from build123d import *

# Parameters (mm, degrees)
F0_W     = 98.428418
F0_H     = 58.695849
F1_DEPTH = 38.1
F2_W     = 23.026837
F2_H     = 29.122172
F3_DEPTH = 37.592
F4_W     = 26.407606
F4_H     = 29.122172
F5_DEPTH = 37.338
F6_W     = 98.428428
F6_H     = 23.929847
F7_DEPTH = 119.888


with BuildPart() as f1:
    # F0 (on Front) → F1 (new body)
    with BuildSketch(Plane.XZ):
        with Locations((-0.45151, 0.225753)):
            Rectangle(F0_W, F0_H)
    extrude(amount=F1_DEPTH)

    # F2 (on face) → F3 (join)
    with BuildSketch(Plane.XZ.offset(38.1)):
        with Locations((-38.1523, -14.561086)):
            Rectangle(F2_W, F2_H)
    extrude(amount=F3_DEPTH)

    # F4 (on face) → F5 (join)
    with BuildSketch(Plane.XZ.offset(38.1)):
        with Locations((35.558896, -14.561086)):
            Rectangle(F4_W, F4_H)
    extrude(amount=F5_DEPTH)

    # F6 (on Front) → F7 (join)
    with BuildSketch(Plane.XZ):
        with Locations((4e-06, -40.635587)):
            Rectangle(F6_W, F6_H)
    extrude(amount=F7_DEPTH)


solid = f1.part
Source: CAD feature listing. Evaluate the final solid. Frame: model axes, mm. A direction names the side the tool comes from. Coordinates: 2 decimals unless noted, no trailing zeros. Loops run counter-clockwise (first coordinate to the right, second up) from the corner with the lowest first, then second, coordinate; pieces in that order, holes last. Notation, with made-up numbers: (-2.5, 55.5) - (14.5, 55.5) arc R11 ccw to (14.5, 62.5) - close; hole circle Ø4 at (43, -11.5). An arc over 180 degrees is marked (long way). One line per question, with ' | ' between items.
1) Section A-A, the plane z = -13. Return loops of the section in (x, y).
Report:
outline: (-49.67, -75.69) - (-26.64, -75.69) - (-26.64, -38.1) - (22.36, -38.1) - (22.36, -75.44) - (48.76, -75.44) - (48.76, 0) - (-49.67, 0) - close
2) Pull-direction query (X, two-part tool) for faces 1 (the face through (-1, -59, -52.601)), 2 (the face through (-26.639, -57, -15)), 3 (the face through (49.214, -59, -41)); classes: released by +X, released by -X, zero draft, split by the parting line, or undercut.
Report:
face 1: zero draft | face 2: undercut | face 3: released by +X
3) Line query: line 1 along X through (y, z) = (-45.5, -10); line 2 along Z through (x, y) = (5, -90.5); line 3 along Y through (x, z) = (15, 20.5). Output: solid intervals per line, ascending.
Report:
line 1: x = -49.67 to -26.64, 22.36 to 48.76 | line 2: z = -52.6 to -28.67 | line 3: y = -38.1 to 0
4) Set-up query: faces 4 (the face through (48.763, -29, -6)), 5 (the face through (35, -75.438, -14)), 6 (the face through (22.355, -57, -15)). Return all of +Z, -Z, +X, -X, +Y, -Y with unobstructed straight access to the full face (end or side cutting, diameter ignored); none if empty.
Report:
face 4: +Z, +X, +Y, -Y | face 5: +Z, +X, -Y | face 6: +Z, -Y
5) Section D-D, the plane x = 4. Return loops of the section in (y, z).
Report:
outline: (-119.89, -52.6) - (0, -52.6) - (0, 29.57) - (-38.1, 29.57) - (-38.1, -28.67) - (-119.89, -28.67) - close
6) First-contact query: P1, Ø14.5, axis at y = -61.5, z = -16, coming from the +X side; P2, Ø18.5, axis at x = -41, y = -51.5, coming from the +Z side; P3, Ø12, axis at x = 34, y = -103, coming from the +Z side. Flat tips, straight axial feed; report the tip coordinate or a pass-through.
Report:
P1: stops at x = 48.76 | P2: stops at z = 0 | P3: stops at z = -28.67
7) Section B-B, the plane x = -35.5. Return loops of the section in (y, z), then the cut area to 3 significant figures.
Report:
outline: (-119.89, -52.6) - (0, -52.6) - (0, 29.57) - (-38.1, 29.57) - (-38.1, 0) - (-75.69, 0) - (-75.69, -28.67) - (-119.89, -28.67) - close | area: 6,170 mm²
8) Section C-C, the plane y = -57.5. Return loops of the section in (x, z).
Report:
outline: (-49.67, -29.12) - (-49.21, -29.12) - (-49.21, -52.6) - (49.21, -52.6) - (49.21, -28.67) - (48.76, -28.67) - (48.76, 0) - (22.36, 0) - (22.36, -28.67) - (-26.64, -28.67) - (-26.64, 0) - (-49.67, 0) - close
